```python
from build123d import *

# Parameters (mm, degrees)
BOSS_EXTRUDE1_DEPTH = 25
SKETCH2_R           = 8.1
CUT_EXTRUDE1_DEPTH  = 49.311489317
SKETCH3_R           = 9.75
CUT_EXTRUDE2_DEPTH  = 8
LPATTERN1_COUNT     = 3
LPATTERN1_PITCH     = 23
FILLET2_R           = 3
BOSS_EXTRUDE2_DEPTH = 10
CHAMFER1_SIZE       = 1.5
FILLET3_R           = 1


with BuildPart() as part:
    # Sketch1 → Boss-Extrude1 (new body)
    with BuildSketch(Plane.XY):
        Polygon((0, 0), (35, 0), (35, 22), (-35, 22), (-35, 0), align=None)
    extrude(amount=BOSS_EXTRUDE1_DEPTH)

    # Sketch2 → Cut-Extrude1 (cut, symmetric)
    with BuildSketch(Plane.XY.offset(25)):
        with Locations((-24, 11)):
            Circle(SKETCH2_R)
    cut_extrude1 = extrude(amount=CUT_EXTRUDE1_DEPTH, both=True, mode=Mode.SUBTRACT)

    # Sketch3 → Cut-Extrude2 (cut)
    with BuildSketch(Plane.XY.offset(25)):
        with Locations((-24, 11)):
            Circle(SKETCH3_R)
    cut_extrude2 = extrude(amount=-CUT_EXTRUDE2_DEPTH, mode=Mode.SUBTRACT)

    # LPattern1: Cut-Extrude1, Cut-Extrude2 ×3
    with Locations(*[(i * LPATTERN1_PITCH, 0, 0) for i in range(1, LPATTERN1_COUNT)]):
        add(cut_extrude1, mode=Mode.SUBTRACT)
        add(cut_extrude2, mode=Mode.SUBTRACT)

    # Fillet2
    # the kernel refuses this fillet: 3 mm, written as the material it takes off along each edge
    with BuildSketch(Plane(origin=(32, 3, 22), x_dir=(1, 0, 0), z_dir=(0, -1, 0))) as fillet2_piece_1_section:
        Polygon((0, 0), (FILLET2_R, 0), (FILLET2_R, FILLET2_R), (0, FILLET2_R), align=None)
    fillet2_piece_1 = extrude(amount=FILLET2_R, mode=Mode.PRIVATE)
    fillet2_piece_1 = fillet2_piece_1 - Plane(origin=(32, 3, 22), x_dir=(-0.7071067811865475, 0, -0.7071067811865475), z_dir=(0, -1, 0)) * Sphere(FILLET2_R, mode=Mode.PRIVATE)
    add(fillet2_piece_1, mode=Mode.SUBTRACT)
    with BuildSketch(Plane(origin=(32, 19, 22), x_dir=(0, 0, 1), z_dir=(1, 0, 0))) as fillet2_piece_2_section:
        Polygon((0, 0), (FILLET2_R, 0), (FILLET2_R, -FILLET2_R), (0, -FILLET2_R), align=None)
    fillet2_piece_2 = extrude(amount=FILLET2_R, mode=Mode.PRIVATE)
    fillet2_piece_2 = fillet2_piece_2 - Plane(origin=(32, 19, 22), x_dir=(0, -0.7071067811865475, -0.7071067811865475), z_dir=(1, 0, 0)) * Sphere(FILLET2_R, mode=Mode.PRIVATE)
    add(fillet2_piece_2, mode=Mode.SUBTRACT)
    with BuildSketch(Plane(origin=(-32, 19, 22), x_dir=(0, 0, 1), z_dir=(-1, 0, 0))) as fillet2_piece_3_section:
        Polygon((0, 0), (FILLET2_R, 0), (FILLET2_R, FILLET2_R), (0, FILLET2_R), align=None)
    fillet2_piece_3 = extrude(amount=FILLET2_R, mode=Mode.PRIVATE)
    fillet2_piece_3 = fillet2_piece_3 - Plane(origin=(-32, 19, 22), x_dir=(0, -0.7071067811865475, -0.7071067811865475), z_dir=(-1, 0, 0)) * Sphere(FILLET2_R, mode=Mode.PRIVATE)
    add(fillet2_piece_3, mode=Mode.SUBTRACT)
    with BuildSketch(Plane(origin=(-32, 3, 22), x_dir=(-1, 0, 0), z_dir=(0, -1, 0))) as fillet2_piece_4_section:
        Polygon((0, 0), (FILLET2_R, 0), (FILLET2_R, -FILLET2_R), (0, -FILLET2_R), align=None)
    fillet2_piece_4 = extrude(amount=FILLET2_R, mode=Mode.PRIVATE)
    fillet2_piece_4 = fillet2_piece_4 - Plane(origin=(-32, 3, 22), x_dir=(0.7071067811865475, 0, -0.7071067811865475), z_dir=(0, -1, 0)) * Sphere(FILLET2_R, mode=Mode.PRIVATE)
    add(fillet2_piece_4, mode=Mode.SUBTRACT)
    with BuildSketch(Plane(origin=(-32, 19, 3), x_dir=(-1, 0, 0), z_dir=(0, 0, -1))) as fillet2_piece_5_section:
        Polygon((0, 0), (FILLET2_R, 0), (FILLET2_R, FILLET2_R), (0, FILLET2_R), align=None)
    fillet2_piece_5 = extrude(amount=FILLET2_R, mode=Mode.PRIVATE)
    fillet2_piece_5 = fillet2_piece_5 - Plane(origin=(-32, 19, 3), x_dir=(0.7071067811865475, -0.7071067811865475, 0), z_dir=(0, 0, -1)) * Sphere(FILLET2_R, mode=Mode.PRIVATE)
    add(fillet2_piece_5, mode=Mode.SUBTRACT)
    with BuildSketch(Plane(origin=(-32, 3, 3), x_dir=(0, 0, -1), z_dir=(0, -1, 0))) as fillet2_piece_6_section:
        Polygon((0, 0), (FILLET2_R, 0), (FILLET2_R, -FILLET2_R), (0, -FILLET2_R), align=None)
    fillet2_piece_6 = extrude(amount=FILLET2_R, mode=Mode.PRIVATE)
    fillet2_piece_6 = fillet2_piece_6 - Plane(origin=(-32, 3, 3), x_dir=(0.7071067811865475, 0, 0.7071067811865475), z_dir=(0, -1, 0)) * Sphere(FILLET2_R, mode=Mode.PRIVATE)
    add(fillet2_piece_6, mode=Mode.SUBTRACT)
    with BuildSketch(Plane(origin=(32, 19, 3), x_dir=(0, 0, -1), z_dir=(1, 0, 0))) as fillet2_piece_7_section:
        Polygon((0, 0), (FILLET2_R, 0), (FILLET2_R, FILLET2_R), (0, FILLET2_R), align=None)
    fillet2_piece_7 = extrude(amount=FILLET2_R, mode=Mode.PRIVATE)
    fillet2_piece_7 = fillet2_piece_7 - Plane(origin=(32, 19, 3), x_dir=(0, -0.7071067811865475, 0.7071067811865475), z_dir=(1, 0, 0)) * Sphere(FILLET2_R, mode=Mode.PRIVATE)
    add(fillet2_piece_7, mode=Mode.SUBTRACT)
    with BuildSketch(Plane(origin=(32, 3, 3), x_dir=(1, 0, 0), z_dir=(0, -1, 0))) as fillet2_piece_8_section:
        Polygon((0, 0), (FILLET2_R, 0), (FILLET2_R, -FILLET2_R), (0, -FILLET2_R), align=None)
    fillet2_piece_8 = extrude(amount=FILLET2_R, mode=Mode.PRIVATE)
    fillet2_piece_8 = fillet2_piece_8 - Plane(origin=(32, 3, 3), x_dir=(-0.7071067811865475, 0, 0.7071067811865475), z_dir=(0, -1, 0)) * Sphere(FILLET2_R, mode=Mode.PRIVATE)
    add(fillet2_piece_8, mode=Mode.SUBTRACT)
    with BuildSketch(Plane(origin=(35, 3, 25), x_dir=(0, 0, -1), z_dir=(0, 1, 0)), Plane(origin=(-35, 19, 25), x_dir=(0, 0, -1), z_dir=(0, -1, 0)), Plane(origin=(-35, 19, 0), x_dir=(1, 0, 0), z_dir=(0, -1, 0))) as fillet2_piece_9:
        with BuildLine():
            CenterArc((FILLET2_R, FILLET2_R), FILLET2_R, 180, 90)
            Line((0, FILLET2_R), (0, 0))
            Line((0, 0), (FILLET2_R, 0))
        make_face()
    extrude(amount=16, mode=Mode.SUBTRACT)
    with BuildSketch(Plane(origin=(32, 22, 25), x_dir=(0, -1, 0), z_dir=(-1, 0, 0)), Plane(origin=(32, 0, 25), x_dir=(0, 0, -1), z_dir=(-1, 0, 0)), Plane(origin=(-32, 0, 0), x_dir=(0, 0, 1), z_dir=(1, 0, 0))) as fillet2_piece_10:
        with BuildLine():
            CenterArc((FILLET2_R, -FILLET2_R), FILLET2_R, 90, 90)
            Line((0, -FILLET2_R), (0, 0))
            Line((0, 0), (FILLET2_R, 0))
        make_face()
    extrude(amount=64, mode=Mode.SUBTRACT)
    with BuildSketch(Plane(origin=(32, 22, 0), x_dir=(0, -1, 0), z_dir=(-1, 0, 0))) as fillet2_piece_11:
        with BuildLine():
            CenterArc((FILLET2_R, FILLET2_R), FILLET2_R, 180, 90)
            Line((0, FILLET2_R), (0, 0))
            Line((0, 0), (FILLET2_R, 0))
        make_face()
    extrude(amount=64, mode=Mode.SUBTRACT)
    with BuildSketch(Plane(origin=(35, 3, 0), x_dir=(0, 0, 1), z_dir=(0, 1, 0))) as fillet2_piece_12:
        with BuildLine():
            CenterArc((FILLET2_R, -FILLET2_R), FILLET2_R, 90, 90)
            Line((0, -FILLET2_R), (0, 0))
            Line((0, 0), (FILLET2_R, 0))
        make_face()
    extrude(amount=16, mode=Mode.SUBTRACT)
    with BuildSketch(Plane(origin=(-35, 0, 3), x_dir=(1, 0, 0), z_dir=(0, 0, 1)), Plane(origin=(-35, 22, 3), x_dir=(0, -1, 0), z_dir=(0, 0, 1))) as fillet2_piece_13:
        with BuildLine():
            CenterArc((FILLET2_R, FILLET2_R), FILLET2_R, 180, 90)
            Line((0, FILLET2_R), (0, 0))
            Line((0, 0), (FILLET2_R, 0))
        make_face()
    extrude(amount=19, mode=Mode.SUBTRACT)
    with BuildSketch(Plane(origin=(35, 22, 3), x_dir=(0, -1, 0), z_dir=(0, 0, 1)), Plane(origin=(35, 0, 3), x_dir=(-1, 0, 0), z_dir=(0, 0, 1))) as fillet2_piece_14:
        with BuildLine():
            CenterArc((FILLET2_R, -FILLET2_R), FILLET2_R, 90, 90)
            Line((0, -FILLET2_R), (0, 0))
            Line((0, 0), (FILLET2_R, 0))
        make_face()
    extrude(amount=19, mode=Mode.SUBTRACT)

    # Sketch5 → Boss-Extrude2 (add)
    with BuildSketch(Plane(origin=(0, 22, 0), x_dir=(1, 0, 0), z_dir=(0, 1, 0))):
        with BuildLine():
            Line((-2.5104146, -8.169868643), (-2.5104146, -4.999995661))
            Line((-2.5104146, -4.999995661), (2.4895854, -4.999995661))
            Line((2.4895854, -4.999995661), (2.4895854, -8.169868643))
            ThreePointArc((2.4895854, -8.169868643), (-0.0104146, -17.499995661), (-2.5104146, -8.169868643))
        make_face()
    extrude(amount=BOSS_EXTRUDE2_DEPTH)

    # Chamfer1
    chamfer1_edges = [part.edges().sort_by_distance(p)[0] for p in [
        (2.4895854, 32, 6.584932152),
        (-0.0104146, 32, 4.999995661),
        (-2.5104146, 32, 6.584932152),
        (-0.0104146, 32, 17.499995661),
    ]]
    chamfer(chamfer1_edges, length=CHAMFER1_SIZE)

    # Fillet3
    fillet3_edges = [part.edges().sort_by_distance(p)[0] for p in [
        (2.4895854, 22, 6.584932152),
        (-0.0104146, 22, 4.999995661),
        (-2.5104146, 22, 6.584932152),
        (-0.0104146, 22, 17.499995661),
    ]]
    fillet(fillet3_edges, radius=FILLET3_R)


solid = part.part
```
CAD build for the part. Positions are in the model's coordinates, mm. A direction names the side the tool comes from. Round coordinates to 2 decimals unless told otherwise and drop trailing zeros. Order: outer loops, then holes, each group sorted by start corner. A loop starts at its lowest first (then second) coordinate and runs counter-clockwise, first axis right, second up. Notation, with made-up numbers: (27, -26.75) - (65, -26.75) arc R20 ccw to (65, 0.25) - close; hole circle Ø1 at (33.25, 43.5). An arc over 180 degrees is marked (long way). Answer in a Markdown table with one row per item. Add a question column.
(1) 3-axis set-ups, long thin cutter, end or side, ignore diameter. For faces 1 (the face through (31.01, 7.27, 21.06)), 2 (the face through (-2.51, 27, 7)), 3 (the face through (0.173, 26.697, 17.497)): which of +Z, -Z, +X, -X, +Y, -Y reach the whole face in a straight line?
(2) Probe L1, parallel to X at y = 11, z = 13.5; L2, parallel to Y at x = -24, z = 19.5; L3, parallel to Y at x = 22, z = 13.75. List the from-to ranges inside material, lowest first. Write a range as [from, to].
(3) Drop flat-ended pins along their axis: pin 1 Ø6 at (x, y) = (-27, 9) entering from +Z; pin 2 Ø1.6 at (y, z) = (27, 6.5) entering from +X; pin 3 Ø1.5 at (x, y) = (-11.5, 21) entering from -Z; pin 4 Ø5.5 at (x, y) = (1, 26) entering from -Z. Give the stop position or say it passes through.
(4) Mould opens along Y. For faces 4 (the face through (0.448, 21.438, 23.748)), 5 (the face through (-13, 11, 25)), 6 (the face through (-26.2, 19, 17)) say: +Y half, -Y half, draft (parallel to the pull), parting line (faces both ways), or undercut.
(5) Band-saw the part on B-B on x = -24. List the corners of the cut face in (y, z).
(6) Band-saw the part on C-C on z = 2.25. List the corners of the cut face in (x, y), and give its area (3 significant figures).
(7) Band-saw the part on D-D on y = 29. List the corners of the cut face in (x, z).
(8) Band-saw the part on A-A on y = 13. Count the separate pieces of the cut face and the enclosed holes in it, and give its area (3 significant figures).
Data:
| question | item | result |
|---|---|---|
| 1 | face 1 | +Z |
| 1 | face 2 | -Z, -X, +Y |
| 1 | face 3 | +Y |
| 2 | L1 | x = [-35, -32.1], [-15.9, -9.1], [7.1, 13.9], [30.1, 35] |
| 2 | L2 | y = [0, 1.25], [20.75, 22] |
| 2 | L3 | y = [0, 2.9], [19.1, 22] |
| 3 | pin 1 | passes through |
| 3 | pin 2 | stops at x = 2.49 |
| 3 | pin 3 | stops at z = 0.27 |
| 3 | pin 4 | stops at z = 5 |
| 4 | face 4 | +Y half |
| 4 | face 5 | draft |
| 4 | face 6 | undercut |
| 5 | outline | (0, 3) arc R3 ccw to (2.9, 0) - (2.9, 17) - (1.25, 17) - (1.25, 24.44) arc R3 ccw to (0, 22) - close; (19.1, 0) arc R3 ccw to (22, 3) - (22, 22) arc R3 ccw to (20.75, 24.44) - (20.75, 17) - (19.1, 17) - close |
| 6 | outline | (-34.9, 3) arc R2.9 ccw to (-32, 0.1) - (32, 0.1) arc R2.9 ccw to (34.9, 3) - (34.9, 19) arc R2.9 ccw to (32, 21.9) - (-32, 21.9) arc R2.9 ccw to (-34.9, 19) - close; hole circle Ø16.2 at (-24, 11); hole circle Ø16.2 at (-1, 11); hole circle Ø16.2 at (22, 11) |
| 6 | area | 897 mm^2 |
| 7 | outline | (-2.51, 5) - (2.49, 5) - (2.49, 8.17) arc R5 ccw (long way) to (-2.51, 8.17) - close |
| 8 | separate pieces | 4 |
| 8 | enclosed holes | 0 |
| 8 | area | 484 mm^2 |
